Design review of the part built by this model. Coordinates are the model's own, in mm. Face numbers are marked on the shaded views. A direction names the side the tool comes from. Coordinates: 2 decimals unless noted, no trailing zeros. Loops run counter-clockwise (first coordinate to the right, second up) from the corner with the lowest first, then second, coordinate; pieces in that order, holes last. Notation, with made-up numbers: (55, 1.25) -> (112, 1.25) arc R14 ccw to (112, 28.25) -> close; hole circle Ø8 at (55, 72). An arc over 180 degrees is marked (long way). Answer as a JSON object with one key per item and string values.
```python
from build123d import *

# Parameters (mm, degrees)
SKETCH1_W           = 16.5
SKETCH1_H           = 16.5
SKETCH1_R           = 1.375
BOSS_EXTRUDE1_DEPTH = 2.5
SKETCH2_R           = 4.25
SKETCH2_R_2         = 1.375
BOSS_EXTRUDE2_DEPTH = 70


with BuildPart() as part:
    # Sketch1 → Boss-Extrude1 (new body)
    with BuildSketch(Plane(origin=(0, 0, 0), x_dir=(1, 0, 0), z_dir=(0, 1, 0))):
        with Locations((0.455521472, -1.417177914)):
            Rectangle(SKETCH1_W, SKETCH1_H)
        with Locations(Location((0.455521472, -1.417177914, 0), (0, 0, 270))):
            Circle(SKETCH1_R, mode=Mode.SUBTRACT)
    extrude(amount=BOSS_EXTRUDE1_DEPTH)

    # Sketch2 → Boss-Extrude2 (add)
    with BuildSketch(Plane(origin=(0, 2.5, 0), x_dir=(1, 0, 0), z_dir=(0, 1, 0))):
        with Locations(Location((0.455521472, -1.417177914, 0), (0, 0, 270))):
            Circle(SKETCH2_R)
        with Locations(Location((0.455521472, -1.417177914, 0), (0, 0, 270))):
            Circle(SKETCH2_R_2, mode=Mode.SUBTRACT)
    extrude(amount=BOSS_EXTRUDE2_DEPTH)


solid = part.part
```
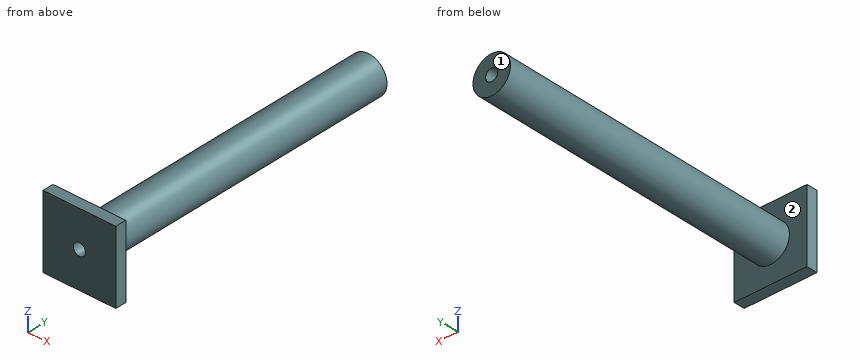
1) Add section D-D, the plane y = 57.5. Give the boundary of the cut face in (x, z) (3 decimals), and give its area (3 significant figures).
Completed:
{"outline": "circle Ø8.5 at (0.456, 1.417); hole circle Ø2.75 at (0.456, 1.417)", "area": "50.8 mm²"}
2) For the marked faces 1 and 2, list the 3-axis set-ups (+Z, -Z, +X, -X, +Y, -Y) from which the entire face can be reached by the end or side of a thin tool; tool diameter is ignored.
Completed:
{"face 1": "+Z, -Z, +X, -X, +Y", "face 2": "+Y"}
3) Add section B-B, the plane x = 3.25. Give the boundary of the cut face in (y, z).
Completed:
{"outline": "(0, -6.83) -> (2.5, -6.83) -> (2.5, -1.78) -> (72.5, -1.78) -> (72.5, 4.62) -> (2.5, 4.62) -> (2.5, 9.67) -> (0, 9.67) -> close"}
4) Add section A-A, the plane z = 1. Give the boundary of the cut face in (x, y) (3 decimals), and give its area (3 significant figures).
Completed:
{"outline": "(-7.794, 0) -> (-0.855, 0) -> (-0.855, 72.5) -> (-3.774, 72.5) -> (-3.774, 2.5) -> (-7.794, 2.5) -> close; (1.766, 0) -> (8.706, 0) -> (8.706, 2.5) -> (4.685, 2.5) -> (4.685, 72.5) -> (1.766, 72.5) -> close", "area": "443 mm²"}
5) Add section C-C, the plane z = 7.25. Give the boundary of the cut face in (x, y), and give its area (4 significant figures).
Completed:
{"outline": "(-7.79, 0) -> (8.71, 0) -> (8.71, 2.5) -> (-7.79, 2.5) -> close", "area": "41.25 mm²"}
6) Clearance check with flat-ended pins moving along their axes: pin 1 Ø5 at (x, y) = (5, 19.5) entering from +Z; pin 2 Ø1 at (x, y) = (-6, 14.5) entering from +Z; pin 3 Ø5 at (y, z) = (56, 0) entering from -X; pin 4 Ø4 at (x, y) = (-2, 15) entering from -Z. State where each tip first meets the part, or that it passes through.
Completed:
{"pin 1": "z = 5.14", "pin 2": "through", "pin 3": "x = -3.79", "pin 4": "z = -2.81"}
7) Wall thickness on probe 1 along Y at (x, z) = (5.25, 4); probe 2 along X at (y, z) = (58, 1.5); probe 3 along Z at (x, y) = (0, 49): over which ranges is each line inside the solid? List them lowest first.
Completed:
{"probe 1": "0 to 2.5", "probe 2": "-3.79 to -0.92, 1.83 to 4.7", "probe 3": "-2.81 to 0.12, 2.71 to 5.64"}
